from build123d import *

# Parameters (mm, degrees)
F2_SIZE  = 1.5
F5_R     = 9
F6_DEPTH = 50


with BuildPart() as f1:
    # F0 (on Front) → F1 (revolve)
    with BuildSketch(Plane.XZ):
        Polygon((0, 66.266628), (-32.55, 66.266628), (-32.55, 43.266628), (-33.25, 43.266628), (-20.2, -75.179155), (-20.2, -106.733372), (0, -106.733372), align=None)
    revolve(axis=Axis((0, 0, -2.596696), (0, 0, -1)))

    # F2
    f2_edges = [f1.edges().sort_by_distance(p)[0] for p in [
        (32.55, 0, 66.266628),
    ]]
    chamfer(f2_edges, length=F2_SIZE)

    # F3 (on Right) → F4 (revolve, cut)
    with BuildSketch(Plane.YZ):
        Polygon((-9, -120), (0, -120), (0, 0), (0, 34.116209), (-9, 34.116209), (-9, 0), align=None)
    revolve(axis=Axis((0, 0, -20.233372), (0, 0, -1)), mode=Mode.SUBTRACT)

    # F5 (on face) → F6 (cut)
    with BuildSketch(Plane.XY.offset(66.266628)):
        with Locations((-15.971139, 10.688378)):
            Circle(F5_R)
        with Locations((17.241976, 8.487223)):
            Circle(F5_R)
        with Locations((-1.270837, -19.175601)):
            Circle(F5_R)
    extrude(amount=-F6_DEPTH, mode=Mode.SUBTRACT)


solid = f1.part
Read the model definition and answer for the solid it produces. Units are mm, in the model's axes. A direction names the side the tool comes from. Round coordinates to 2 decimals unless told otherwise and drop trailing zeros. Write each loop counter-clockwise with the first axis right and the second up, starting at its lowest first coordinate (ties: lowest second). Pieces come first, ordered by that corner, then holes.
1. The part is cut by section A-A, the plane z = -33. Determine the outline of the cut face in (x, y), then the cut area to 3 significant figures.
2. Given pin 1 Ø20.5 at (x, y) = (0, 0) entering from -Z; pin 2 Ø5 at (y, z) = (17.5, -69) entering from -X; pin 3 Ø14.5 at (x, y) = (17.24, 8.49) entering from +Z; pin 4 Ø3 at (x, z) = (25, 30.5) entering from -Y, each flat-ended and moving along its own axis, determine where each tip first touches the part or whether it passes through.
3. The part is cut by section C-C, the plane z = 55. Determine the outline of the cut face in (x, y), then the cut area to 3 significant figures.
4. Which of the six approach directions +Z, -Z, +X, -X, +Y, -Y give full straight-line access (tool end or side, diameter ignored) to faces 1 (the face through (0, 0, 66.267)), 2 (the face through (0, 0, 34.116)), 3 (the face through (22, -24.5, 43.267))?
5. The part is cut by section B-B, the plane x = 0. Determine the outline of the cut face in (y, z).
6. Straight lines are drawn through the part: L1, parallel to X at y = 3, z = 33.5; L2, parallel to Y at x = 0, z = -75; L3, parallel to Y at x = -8, z = 39. For each, find the intervals that lie inside material, in ascending order.
7. The part is cut by section D-D, the plane z = 5.5. Determine the outline of the cut face in (x, y), then the cut area to 3 significant figures.
8. Determine the mould class of faces 4 (the face through (-9, -4, -106.733)), 5 (the face through (-16, 11, 16.267)), 6 (the face through (25.83, -19.81, 53.87)) for opening direction Y: pulls with the +Y half, pulls with the -Y half, needs draft (parallel to the pull), parting line crosses it, or undercut.
Values:
1. outline: circle Ø49.69 at (0, 0); hole circle Ø18 at (0, 0)
1. area: 1,690 mm2
2. pin 1: stops at z = -106.73
2. pin 2: stops at x = -14.56
2. pin 3: stops at z = 16.27
2. pin 4: stops at y = -21.51
3. outline: circle Ø65.1 at (0, 0); hole circle Ø18 at (-15.97, 10.69); hole circle Ø18 at (-1.27, -19.18); hole circle Ø18 at (17.24, 8.49)
3. area: 2,570 mm2
4. face 1: +Z, +X, -X, +Y, -Y
4. face 2: -Z
4. face 3: +Z
5. outline: (-33.25, 43.27) - (-20.2, -75.18) - (-20.2, -106.73) - (-9, -106.73) - (-9, 34.12) - (9, 34.12) - (9, -106.73) - (20.2, -106.73) - (20.2, -75.18) - (33.25, 43.27) - (32.55, 43.27) - (32.55, 64.77) - (31.05, 66.27) - (-10.27, 66.27) - (-10.27, 16.27) - (-28.09, 16.27) - (-28.09, 66.27) - (-31.05, 66.27) - (-32.55, 64.77) - (-32.55, 43.27) - close
6. L1: x = -32.03 to -20.65, -11.29 to -8.49, 8.49 to 10.11, 24.38 to 32.03
6. L2: y = -20.22 to -9, 9 to 20.22
6. L3: y = -31.79 to -25.15, -13.2 to 6.51, 14.87 to 31.79
7. outline: circle Ø58.18 at (0, 0); hole circle Ø18 at (0, 0)
7. area: 2,400 mm2
8. face 4: needs draft
8. face 5: undercut
8. face 6: parting line crosses it
